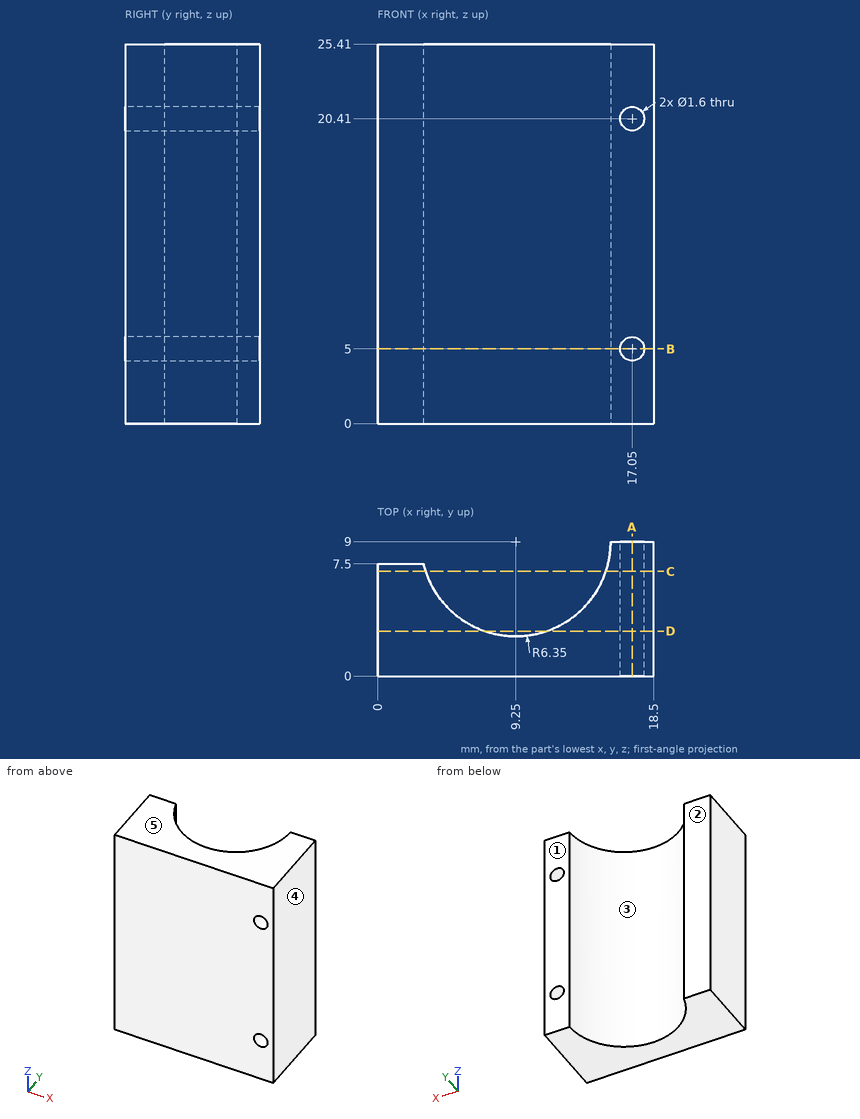
The drawing under review shows one solid part. Ordinate dimensions are in mm from its lowest x, y, z. A direction names the side the tool comes from. Round coordinates to 2 decimals unless told otherwise and drop trailing zeros. Order: outer loops, then holes, each group sorted by start corner. A loop starts at its lowest first (then second) coordinate and runs counter-clockwise, first axis right, second up. Notation, with made-up numbers: (-26, 10) -> (30, 10) arc R27 ccw to (30, 34) -> close; hole circle Ø11 at (-30.5, 28). An arc over 180 degrees is marked (long way). Use a Markdown table: item, result.
Q1. We need section A-A on x = 17.05. Write out the cut boundary in (y, z), then the cut area to 3 significant figures.
Values:
| item | result |
|---|---|
| outline | (0, 0) -> (9, 0) -> (9, 4.2) -> (0, 4.2) -> close; (0, 5.8) -> (9, 5.8) -> (9, 19.61) -> (0, 19.61) -> close; (0, 21.21) -> (9, 21.21) -> (9, 25.41) -> (0, 25.41) -> close |
| area | 200 mm^2 |
Q2. Tool access review of the marked faces 1 and 2: name each direction out of +Z, -Z, +X, -X, +Y, -Y from which nothing blocks a thin tool from reaching the whole face with its end or side.
Values:
| item | result |
|---|---|
| face 1 | +Z, -Z, +X, -X, +Y |
| face 2 | +Z, -Z, -X, +Y |
Q3. Mouldability with a two-part tool opening along X and no side actions: class the marked faces 3, 4 and 5 as +X half, -X half, draft (parallel to the pull), parting line (faces both ways), or undercut.
Values:
| item | result |
|---|---|
| face 3 | undercut |
| face 4 | +X half |
| face 5 | draft |
Q4. We need section D-D on y = 3. Write out the cut boundary in (x, z).
Values:
| item | result |
|---|---|
| outline | (0, 0) -> (7.17, 0) -> (7.17, 25.41) -> (0, 25.41) -> close; (11.33, 0) -> (18.5, 0) -> (18.5, 25.41) -> (11.33, 25.41) -> close; hole circle Ø1.6 at (17.05, 5); hole circle Ø1.6 at (17.05, 20.41) |
Q5. For line 1 (X direction, y = 7.25, z = 20.41); line 2 (X direction, y = 2, z = 5); line 3 (X direction, y = 4, z = 5), list the stretches that pass through material, from the lowest coordinate up.
Values:
| item | result |
|---|---|
| line 1 | x = 0 to 3.15, 15.35 to 16.25, 17.85 to 18.5 |
| line 2 | x = 0 to 16.25, 17.85 to 18.5 |
| line 3 | x = 0 to 5.34, 13.16 to 16.25, 17.85 to 18.5 |
Q6. We need section C-C on y = 7. Write out the cut boundary in (x, z), then the cut area to 3 significant figures.
Values:
| item | result |
|---|---|
| outline | (0, 0) -> (3.22, 0) -> (3.22, 25.41) -> (0, 25.41) -> close; (15.28, 0) -> (18.5, 0) -> (18.5, 25.41) -> (15.28, 25.41) -> close; hole circle Ø1.6 at (17.05, 5); hole circle Ø1.6 at (17.05, 20.41) |
| area | 160 mm^2 |
Q7. We need section B-B on z = 5. Write out the cut boundary in (x, y).
Values:
| item | result |
|---|---|
| outline | (0, 0) -> (16.25, 0) -> (16.25, 9) -> (15.6, 9) arc R6.35 cw to (3.08, 7.5) -> (0, 7.5) -> close; (17.85, 0) -> (18.5, 0) -> (18.5, 9) -> (17.85, 9) -> close |
Q8. Clearance check with flat-ended pins moving along their axes: P1, Ø2, axis at x = 7, z = 20, coming from the +Y side; P2, Ø1.5, axis at x = 2, z = 19, coming from the +Y side; P3, Ø1.3, axis at x = 17.05, z = 5, coming from the -Y side; P4, Ø3, axis at x = 11.5, z = 21.5, coming from the +Y side. State where each tip first meets the part, or that it passes through.
Values:
| item | result |
|---|---|
| P1 | stops at y = 3.54 |
| P2 | stops at y = 7.5 |
| P3 | passes through |
| P4 | stops at y = 3.88 |
